The listing builds one solid part. Answer for the finished solid, in the listing's coordinates (mm). A direction names the side the tool comes from. Give positions to 0.01 mm unless a question says otherwise; leave off trailing zeros. Write each loop counter-clockwise with the first axis right and the second up, starting at its lowest first coordinate (ties: lowest second). Pieces come first, ordered by that corner, then holes. Notation, with made-up numbers: (18.25, 8.5) -> (29.25, 8.5) arc R7 cw to (29.25, 16.5) -> close; hole circle Ø11 at (22.25, 79). An arc over 180 degrees is marked (long way). Put each result on its own line as item: value. Start each with the question number.
1) A cutting plane is placed at C-C (y = 36). Write down the section's boundary in (x, z), then the cut area to 3 significant figures.
2) For a pull along Y with two mould halves and no side action, classify faces 5 (the flat face through (0.84, 81.887, 4.555)), 6 (the flat face through (-55, -30, 5)), 7 (the flat face through (-60, 0, 36)) as released by +Y, released by -Y, zero draft, split by the parting line, or undercut.
3) Flat-ended cylindrical pins translate along their axes: pin 1 Ø5 at (x, y) = (-57, -31.5) entering from +Z; pin 2 Ø11 at (x, y) = (56, -40) entering from +Z; pin 3 Ø3 at (x, y) = (52.5, 17.5) entering from +Z; pin 4 Ø6 at (x, y) = (-19.5, 38.5) entering from -Z. Find the tip coordinate at first contact, or state that the pin passes through.
4) Find the intervals of material crossed by line 1 along Y through (x, z) = (-30.5, 13.5); line 2 along Z through (x, y) = (53, -76.5); line 3 along X through (y, z) = (4.5, 88), in increasing order. Write a range as from..to.
5) A cutting plane is placed at B-B (z = 86). Write down the section's boundary in (x, y), then the cut area to 3 significant figures.
6) For faces 1 (the flat face through (-1, 41.58, 14)), 2 (the flat face through (0.84, 73.98, 3.576)), 3 (the flat face through (54.9, -6.6, 14.9)), 4 (the flat face through (-46.04, -0.32, 50.71)), determine the directions among +Z, -Z, +X, -X, +Y, -Y from which every point of the face is accessible in a straight line to the end or side of a thin tool.
7) A cutting plane is placed at A-A (x = -7). Give the number of separate pieces and of enclosed holes in the cut face, then the cut area to 3 significant figures.
from build123d import *

# Parameters (mm, degrees)
F1_DEPTH   = 60
F3_DEPTH   = 25
F4_W       = 100
F4_H       = 41.5797430669
F5_DEPTH   = 30.001
F5_FACE_W  = 100
F5_FACE_H  = 5
F6_REACH   = 142.3730132293
F5_FACE1_W = 100
F5_FACE1_H = 5
F7_REACH   = 142.3730132293


with BuildPart() as f1:
    # F0 (on Right) → F1 (new body, symmetric)
    with BuildSketch(Plane.YZ):
        with BuildLine():
            Line((-80, 0), (0, 0))
            Line((0, 0), (80, 0))
            Line((80, 0), (83.8268343237, 9.2387953251))
            Line((83.8268343237, 9.2387953251), (81.9790752586, 10.0041621898))
            Line((81.9790752586, 10.0041621898), (78.5349243673, 1.6892463972))
            Line((78.5349243673, 1.6892463972), (69.2961290422, 5.5160807209))
            Line((69.2961290422, 5.5160807209), (66.5901485415, 12.0488955453))
            Line((66.5901485415, 12.0488955453), (64.6767313797, 7.4294978827))
            Line((64.6767313797, 7.4294978827), (55.4379360546, 11.2563322064))
            Line((55.4379360546, 11.2563322064), (52.7319555538, 17.7891470308))
            Line((52.7319555538, 17.7891470308), (50.818538392, 13.1697493682))
            Line((50.818538392, 13.1697493682), (41.5797430669, 16.9965836918))
            ThreePointArc((41.5797430669, 16.9965836918), (19.6436139822, 34.3018638475), (10, 60.5252730432))
            Line((10, 60.5252730432), (4.9851213736, 125.3854411629))
            ThreePointArc((4.9851213736, 125.3854411629), (3.3965272107, 128.6692782543), (0, 130))
            ThreePointArc((0, 130), (-3.3965272107, 128.6692782543), (-4.9851213736, 125.3854411629))
            Line((-4.9851213736, 125.3854411629), (-10, 60.5252730432))
            ThreePointArc((-10, 60.5252730432), (-19.6436139822, 34.3018638475), (-41.5797430669, 16.9965836918))
            Line((-41.5797430669, 16.9965836918), (-50.818538392, 13.1697493682))
            Line((-50.818538392, 13.1697493682), (-52.7319555538, 17.7891470308))
            Line((-52.7319555538, 17.7891470308), (-55.4379360546, 11.2563322064))
            Line((-55.4379360546, 11.2563322064), (-64.6767313797, 7.4294978827))
            Line((-64.6767313797, 7.4294978827), (-66.5901485415, 12.0488955453))
            Line((-66.5901485415, 12.0488955453), (-69.2961290422, 5.5160807209))
            Line((-69.2961290422, 5.5160807209), (-78.5349243673, 1.6892463972))
            Line((-78.5349243673, 1.6892463972), (-81.9790752586, 10.0041621898))
            Line((-81.9790752586, 10.0041621898), (-83.8268343237, 9.2387953251))
            Line((-83.8268343237, 9.2387953251), (-80, 0))
        make_face()
        Polygon((-10.5511115466, 24.437102688), (-2.5, 5), (-57.4764284691, 5), align=None, mode=Mode.SUBTRACT)
        Polygon((57.4764284691, 5), (2.5, 5), (10.5511115466, 24.437102688), align=None, mode=Mode.SUBTRACT)
    extrude(amount=F1_DEPTH, both=True)

    # F2 (on Front) → F3 (cut, symmetric)
    with BuildSketch(Plane.XZ):
        with BuildLine():
            ThreePointArc((0, 115.3854411629), (-25.9524271926, 106.0449266507), (-40, 82.3080484491))
            Line((-40, 82.3080484491), (-50, 30))
            Line((-50, 30), (0, 30))
            Line((0, 30), (50, 30))
            Line((50, 30), (40, 82.3080484491))
            ThreePointArc((40, 82.3080484491), (25.9524271926, 106.0449266507), (0, 115.3854411629))
        make_face()
    extrude(amount=F3_DEPTH, both=True, mode=Mode.SUBTRACT)

    # F4 (on face) → F5 (cut, through all)
    with BuildSketch(Plane.XY.offset(30)):
        with Locations((0, 20.7898715334)):
            Rectangle(F4_W, F4_H)
        with Locations((0, -20.7898715334)):
            Rectangle(F4_W, F4_H)
    extrude(amount=-F5_DEPTH, mode=Mode.SUBTRACT)

    f6_end = Plane(origin=(0, 43.7688782858, 10.6778531928), x_dir=(0, -0.9238795325, 0.3826834324), z_dir=(0, -0.3826834324, -0.9238795325))
    # F5_face (on face) → F6 (cut, up to a plane its end follows)
    with BuildSketch(Plane(origin=(0, 41.5797430669, 2.5), x_dir=(1, 0, 0), z_dir=(0, -1, 0))):
        Rectangle(F5_FACE_W, F5_FACE_H)
    f6_long = extrude(amount=-F6_REACH, mode=Mode.PRIVATE)
    add(split(f6_long, bisect_by=f6_end, keep=Keep.TOP, mode=Mode.PRIVATE), mode=Mode.SUBTRACT)

    f7_end = Plane(origin=(0, -43.7688782858, 10.6778531928), x_dir=(0, -0.9238795325, -0.3826834324), z_dir=(0, 0.3826834324, -0.9238795325))
    # F5_face1 (on face) → F7 (cut, up to a plane its end follows)
    with BuildSketch(Plane(origin=(0, -41.5797430669, 2.5), x_dir=(-1, 0, 0), z_dir=(0, 1, 0))):
        Rectangle(F5_FACE1_W, F5_FACE1_H)
    f7_long = extrude(amount=-F7_REACH, mode=Mode.PRIVATE)
    add(split(f7_long, bisect_by=f7_end, keep=Keep.TOP, mode=Mode.PRIVATE), mode=Mode.SUBTRACT)


solid = f1.part
Reply:
1. outline: (-60, 0) -> (-50, 0) -> (-50, 5) -> (-60, 5) -> close; (-60, 13.9) -> (-50, 13.9) -> (-50, 19.71) -> (-60, 19.71) -> close; (50, 0) -> (60, 0) -> (60, 5) -> (50, 5) -> close; (50, 13.9) -> (60, 13.9) -> (60, 19.71) -> (50, 19.71) -> close
1. area: 216 mm2
2. face 5: released by +Y
2. face 6: undercut
2. face 7: zero draft
3. pin 1: stops at z = 24.46
3. pin 2: stops at z = 20.59
3. pin 3: stops at z = 40.1
3. pin 4: passes through
4. line 1: y = -54.51..-50.96, -50.02..-41.58, 41.58..50.02, 50.96..54.51
4. line 2: z = 0..2.53
4. line 3: x = -60..-38.48, 38.48..60
5. outline: (-60, -8.03) -> (-39.11, -8.03) -> (-39.11, 8.03) -> (-60, 8.03) -> close; (39.11, -8.03) -> (60, -8.03) -> (60, 8.03) -> (39.11, 8.03) -> close
5. area: 671 mm2
6. face 1: +Z, -Z
6. face 2: +Z, +X, -X
6. face 3: +X, -X
6. face 4: -Z, +Y, -Y
7. separate pieces: 3
7. enclosed holes: 0
7. area: 607 mm2
